Answer from the drawing. Dimensions are ordinates in mm from the lowest x, y and z of the part. A direction names the side the tool comes from. Give positions to 0.01 mm unless a question says otherwise; leave off trailing zeros. Order: outer loops, then holes, each group sorted by start corner. A loop starts at its lowest first (then second) coordinate and runs counter-clockwise, first axis right, second up.
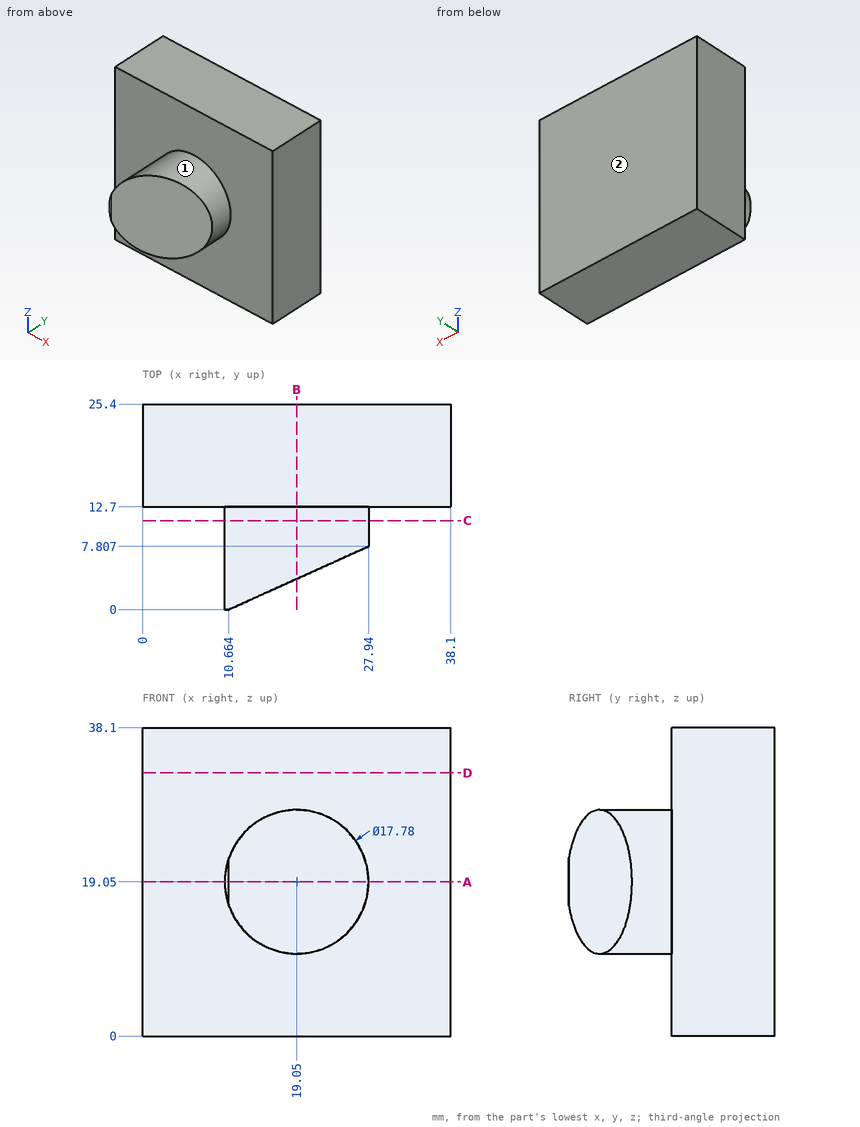
1) The part is cut by section D-D on z = 32.5. Determine the outline of the cut face in (x, y), and give its area (3 significant figures).
Final values:
outline: (0, 12.7) - (38.1, 12.7) - (38.1, 25.4) - (0, 25.4) - close
area: 484 mm2
2) Given pin 1 (3 mm diameter, centred on y = 3, z = 24.5, fed in from +X); pin 2 (3 mm diameter, centred on x = 13.5, y = 8, fed in from +Z); pin 3 (3 mm diameter, centred on x = 28, z = 31, fed in from -Y); pin 4 (4 mm diameter, centred on y = 14.5, z = 10, fed in from -X), each flat-ended and moving along its own axis, determine where each tip first touches the part or whether it passes through.
Final values:
pin 1: stops at x = 20.62
pin 2: stops at z = 26.96
pin 3: stops at y = 12.7
pin 4: stops at x = 0
3) The part is cut by section C-C on y = 11. Determine the outline of the cut face in (x, z).
Final values:
outline: circle Ø17.78 at (19.05, 19.05)
4) The part is cut by section A-A on z = 19.05. Determine the outline of the cut face in (x, y).
Final values:
outline: (0, 12.7) - (10.16, 12.7) - (10.16, 0) - (10.66, 0) - (27.94, 7.81) - (27.94, 12.7) - (38.1, 12.7) - (38.1, 25.4) - (0, 25.4) - close
5) A tool of negligible diameter and unlimited length cuts with its end or side. For the marked faces 1 and 2, from which of +Z, -Z, +X, -X, +Y, -Y can it reach the whole face along a straight path? Write none if from no direction.
Final values:
face 1: -Y
face 2: +Z, -Z, +X, -X, +Y
6) The part is cut by section B-B on x = 19.05. Determine the outline of the cut face in (y, z), and give its area (3 significant figures).
Final values:
outline: (3.79, 10.16) - (12.7, 10.16) - (12.7, 0) - (25.4, 0) - (25.4, 38.1) - (12.7, 38.1) - (12.7, 27.94) - (3.79, 27.94) - close
area: 642 mm2
7) Consider L1, parallel to Y at x = 11.5, z = 34.5; L2, parallel to Y at x = 26, z = 22; L3, parallel to X at y = 5.5, z = 22.5 (1 decimal). Determine where each line is inside the solid, lowest interval first.
Final values:
L1: y = 12.7 to 25.4
L2: y = 6.93 to 25.4
L3: x = 10.9 to 22.8
